Geometry: final body of the model. Coordinates: model frame, mm. Face numbers are marked on the shaded views. A direction names the side the tool comes from. Give positions to 0.01 mm unless a question says otherwise; leave off trailing zeros. Loops run counter-clockwise (first coordinate to the right, second up) from the corner with the lowest first, then second, coordinate; pieces in that order, holes last. Notation, with made-up numbers: (-1, 85.25) -> (13, 85.25) arc R15 ccw to (13, 99.25) -> close; hole circle Ø10 at (56, -12). An arc over 180 degrees is marked (long way). One line per question, with ' | ' between items. Start each with the question number.
Item 1: Section D-D on z = 9.5. Return loops of the section in (x, y).
Item 2: Material intervals for line 1 along Y through (x, z) = (0, 15.25); line 2 along Y through (x, z) = (-2, 14.5); line 3 along Y through (x, z) = (1.25, 3.25), sorted ascending. Write a range as [from, to].
Item 3: Section A-A on y = 0. Return loops of the section in (x, z), then the cut area to 3 significant figures.
Item 4: Pin query (flat end, axial travel): P1, Ø0.9, axis at x = -0.5, y = -0.5, coming from the -Z side; P2, Ø1, axis at y = -2.5, z = 14.5, coming from the -X side; P3, Ø2, axis at y = 2, z = 12.5, coming from the +X side. Return the tip coordinate at first contact, or that it passes through.
Item 5: Set-up query: the marked faces 1 and 2. Return all of +Z, -Z, +X, -X, +Y, -Y with unobstructed straight access to the full face (end or side cutting, diameter ignored); none if empty.
Item 6: Section C-C on z = 4. Return loops of the section in (x, y).
Autodesk Fusion 360 part; units mm, degrees
sketch "スケッチ1" plane through (0, 0, 0) normal (0, 0, 1) x (1, 0, 0)
  circle A0 centre (0, 0) radius 4
  dimension "d1" = 8
extrude "押し出し1" add sketch "スケッチ1" along normal blind 19
cylinder "円柱プリミティブ1" cut diameter 2 height -5 placed x (1, 0, 0) y (0, 1, 0) z (0, 0, 1) at (0, 0, 19)
thread "ねじ1" thread offset 0 thread length 10
cylinder "円柱プリミティブ2" cut diameter 3 height -5 placed x (0, 1, 0) y (1, 0, 0) z (0, 0, -1) at (0, 0, 0)
thread "ねじ2" thread offset 0 thread length 10
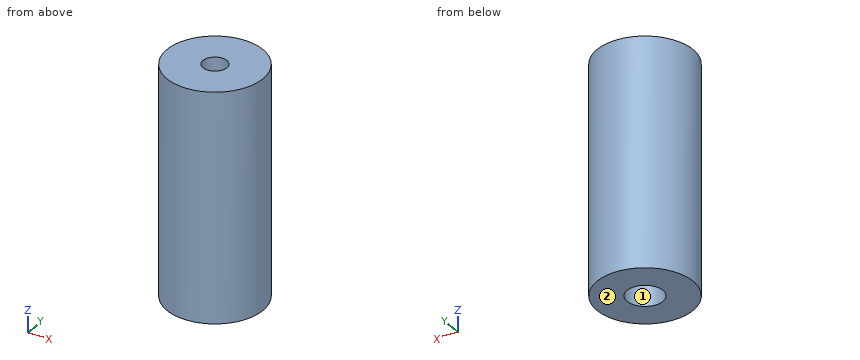
Result sheet:
1) outline: circle Ø8 at (0, 0)
2) line 1: y = [-4, -1], [1, 4] | line 2: y = [-3.46, 3.46] | line 3: y = [-3.8, -0.83], [0.83, 3.8]
3) outline: (-4, 0) -> (-1.5, 0) -> (-1.5, 5) -> (1.5, 5) -> (1.5, 0) -> (4, 0) -> (4, 19) -> (1, 19) -> (1, 14) -> (-1, 14) -> (-1, 19) -> (-4, 19) -> close | area: 127 mm²
4) P1: stops at z = 5 | P2: stops at x = -3.46 | P3: stops at x = 3.87
5) face 1: -Z | face 2: -Z, +X, -X, +Y, -Y
6) outline: circle Ø8 at (0, 0); hole circle Ø3 at (0, 0)
